Autodesk Inventor part; units mm, degrees
ref_plane "YZ Plane" through (0, 0, 0) normal (1, 0, 0) x (0, 1, 0)
ref_plane "XZ Plane" through (0, 0, 0) normal (0, 1, 0) x (-1, 0, 0)
ref_plane "XY Plane" through (0, 0, 0) normal (0, 0, 1) x (1, 0, 0)
sketch "Sketch1" plane through (0, 0, 0) normal (0, 1, 0) x (-1, 0, 0)
  line L0 (-11, 20) -> (11, 20)
  line L1 (11, 20) -> (11, -20)
  line L2 (11, -20) -> (-11, -20)
  line L3 (-11, -20) -> (-11, 20)
  line L4 (-11, 20) -> (11, -20) construction
  line L5 (11, 20) -> (-11, -20) construction
  line L6 (-11, -20) -> (-11, -12)
  line L7 (-11, 20) -> (-11, 9)
  line L8 (0, -20) -> (0, -12)
  line L9 (0, 20) -> (0, 8)
  line L10 (-4.6188, 0) -> (-9.2376, 8)
  line L11 (-9.2376, 8) -> (-4.6188, 16)
  line L12 (-4.6188, 16) -> (4.6188, 16)
  line L13 (4.6188, 16) -> (9.2376, 8)
  line L14 (9.2376, 8) -> (4.6188, 0)
  line L15 (4.6188, 0) -> (-4.6188, 0)
  dimension "d0" = 22
  dimension "d1" = 40
  dimension "d35" = 12
  dimension "d36" = 16
extrude "Plate1" add sketch "Sketch1" along normal blind 4.7 contours L0 L1 L2 L3 | L10 L11 L12 L13 L14 L15
hole "Hole4" at (0, 0, -12) direction (0, 1, 0) diameter 9 end through all
full round fillet "Fillet2" first side at (11, 1.5667, 6.6667) centre faces at (3.6667, 3.1333, -20) second side at (-11, 1.5667, -6.6667)
extrude "Cut1" cut sketch "Sketch1" along normal blind 4.7 contours L10 L11 L12 L13 L14 L15
equation "\"d31\" = Thickness"
equation "\"d37\" = Thickness"
equation "\"d3\" = Thickness"
equation "\"BendRadius\" = Thickness"
equation "\"BendReliefWidth\" = Thickness"
equation "\"BendReliefDepth\" = 0.5 * Thickness"
equation "\"CornerReliefSize\" = 4 * Thickness"
equation "\"MinimumRemnant\" = 2 * Thickness"
equation "\"TransitionRadius\" = BendRadius"
equation "\"JacobiRadiusSize\" = BendRadius"
equation "\"GapSize\" = Thickness"
properties part number "chapa"
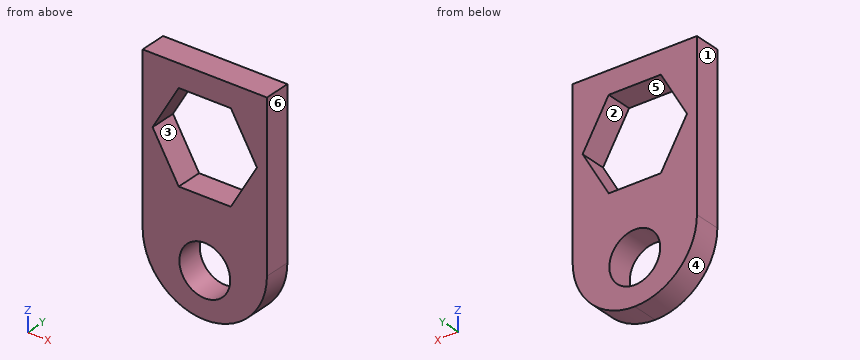
Source: CAD feature listing. Evaluate the final solid. Frame: model axes, mm. Face numbers are marked on the shaded views. A direction names the side the tool comes from. Round coordinates to 2 decimals unless told otherwise and drop trailing zeros. Loops run counter-clockwise (first coordinate to the right, second up) from the corner with the lowest first, then second, coordinate; pieces in that order, holes last. Notation, with made-up numbers: (41.25, -32.75) - (47.25, -32.75) arc R28 ccw to (47.25, -10.75) - close; hole circle Ø1 at (53, 35.5). An arc over 180 degrees is marked (long way). Write item = value, one per line. Start each with the question number.
Item 1: Reachability of the marked faces 5 and 6 from +Z, -Z, +X, -X, +Y, -Y: full face, straight path, thin tool, end or side. Return the list, or none.
Item 2: Section query B-B on z = 3. Output: boundary loops of the cut face in (x, y).
Item 3: Section query A-A on y = 1.85. Count the separate pieces of the cut face and the enclosed holes in it, plus the area to 3 significant figures.
Item 4: Mould query, pull axis Z, two halves, no side actions, for the marked faces 1, 2, 3 and 4. Classes: released by +Z, released by -Z, zero draft, split by the parting line, or undercut.
Item 5: Material intervals for line 1 (Z direction, x = 0, y = 2.2); line 2 (Z direction, x = 1.75, y = 3.6); line 3 (Z direction, x = -8.5, y = 3.85), sorted ascending.
Item 6: First-contact query: pin 1 Ø1.5 at (x, y) = (1.5, 4) entering from -Z; pin 2 Ø1.5 at (x, y) = (3, 2.5) entering from -Z; pin 3 Ø10.5 at (x, z) = (0, -12) entering from -Y; pin 4 Ø2 at (x, y) = (-3.5, 2.5) entering from -Z. Flat tips, straight axial feed; report the tip coordinate or a pass-through.
Item 7: Section query D-D on x = 7.75. Output: boundary loops of the cut face in (y, z), plus the area to 3 significant figures.
Item 8: Section query C-C on x = 4. Output: boundary loops of the cut face in (y, z).
Results list:
q1.face_5 = +Y, -Y
q1.face_6 = +Z, -Z, +X, +Y, -Y
q2.outline = (-11, 0) - (-6.35, 0) - (-6.35, 4.7) - (-11, 4.7) - close; (6.35, 0) - (11, 0) - (11, 4.7) - (6.35, 4.7) - close
q3.separate_pieces = 1
q3.enclosed_holes = 2
q3.area = 543 mm²
q4.face_1 = zero draft
q4.face_2 = undercut
q4.face_3 = undercut
q4.face_4 = released by -Z
q5.line_1 = -20 to -16.5, -7.5 to 0, 16 to 20
q5.line_2 = -19.86 to -16.15, -7.85 to 0, 16 to 20
q5.line_3 = -15.98 to 6.72, 9.28 to 20
q6.pin_1 = -19.97
q6.pin_2 = -19.77
q6.pin_3 = 0
q6.pin_4 = -19.71
q7.outline = (0, -16.81) - (4.7, -16.81) - (4.7, 5.42) - (0, 5.42) - close; (0, 10.58) - (4.7, 10.58) - (4.7, 20) - (0, 20) - close
q7.area = 149 mm²
q8.outline = (0, -19.25) - (4.7, -19.25) - (4.7, -14.06) - (0, -14.06) - close; (0, -9.94) - (4.7, -9.94) - (4.7, 0) - (0, 0) - close; (0, 16) - (4.7, 16) - (4.7, 20) - (0, 20) - close
